```python
from build123d import *

# Parameters (mm, degrees)
RESSALTO_EXTRUS_O1_DEPTH = 20
CORTE_EXTRUS_O1_DEPTH    = 118
CORTE_EXTRUS_O2_DEPTH    = 137.674796506
ESBO_O4_R                = 11.969366969
CORTE_EXTRUS_O3_DEPTH    = 137.674796506


with BuildPart() as part:
    # Esboço1 → Ressalto-extrusão1 (new body)
    with BuildSketch(Plane.XY):
        Polygon((0, 0), (0, 18), (8, 18), (8, 8), (126, 8), (126, 18), (134, 18), (134, 0), align=None)
    extrude(amount=RESSALTO_EXTRUS_O1_DEPTH)

    # Esboço2 → Corte-extrusão1 (cut)
    with BuildSketch(Plane(origin=(8, 0, 0), x_dir=(0, 0, -1), z_dir=(1, 0, 0))):
        with BuildLine():
            Line((-20, 8), (0, 8))
            ThreePointArc((0, 8), (-10, 6.284271247), (-20, 8))
        make_face()
    extrude(amount=CORTE_EXTRUS_O1_DEPTH, mode=Mode.SUBTRACT)

    # Esboço3 → Corte-extrusão2 (cut, through all)
    with BuildSketch(Plane(origin=(0, 0, 0), x_dir=(-1, 0, 0), z_dir=(0, 0, -1))):
        with BuildLine():
            Line((-8, 18), (-7.073837994, 18))
            ThreePointArc((-7.073837994, 18), (-7.767965092, 13.021398611), (-8, 8))
            Line((-8, 8), (-8, 18))
        make_face()
        with BuildLine():
            Line((-126, 8), (-126, 18))
            Line((-126, 18), (-126.926162006, 18))
            ThreePointArc((-126.926162006, 18), (-126.232034908, 13.021398611), (-126, 8))
        make_face()
    extrude(amount=-CORTE_EXTRUS_O2_DEPTH, mode=Mode.SUBTRACT)

    # Esboço4 → Corte-extrusão3 (cut, through all)
    with BuildSketch(Plane.ZY):
        with Locations((10, 27.253795072)):
            Circle(ESBO_O4_R)
    extrude(amount=-CORTE_EXTRUS_O3_DEPTH, mode=Mode.SUBTRACT)


solid = part.part
```
Input: part model. Units: mm. Frame: model coordinates. A direction names the side the tool comes from. Give positions to 0.01 mm unless a question says otherwise; leave off trailing zeros. Write each loop counter-clockwise with the first axis right and the second up, starting at its lowest first coordinate (ties: lowest second). Pieces come first, ordered by that corner, then holes. Notation, with made-up numbers: (-22, 47.5) - (16, 47.5) arc R29 ccw to (16, 84.5) - close; hole circle Ø8 at (85.25, 54). An arc over 180 degrees is marked (long way). Write item = value, one per line. Start each with the question number.
1) Draft query along X for faces 1 (the face through (0, 9, 10)), 2 (the face through (134, 9, 10)), 3 (the face through (126.146, 11.978, 9.86)), 4 (the face through (68, 5, 20)). Return one class per face: pulls with the +X half, pulls with the -X half, needs draft (parallel to the pull), parting line crosses it, or undercut.
2) Pin query (flat end, axial travel): pin 1 (4 mm diameter, centred on x = 101, z = 17.5, fed in from +Y); pin 2 (6 mm diameter, centred on y = 6.5, z = 15.5, fed in from -X); pin 3 (12 mm diameter, centred on x = 20, z = 16.5, fed in from +Y). Return the tip coordinate at first contact, or that it passes through.
3) Reachability of faces 5 (the face through (130.192, 15.285, 9.885)), 6 (the face through (7.854, 11.978, 9.86)), 7 (the face through (66.174, 6.285, 9.857)) from +Z, -Z, +X, -X, +Y, -Y: full face, straight path, thin tool, end or side. Return the list, or none.
4) Material intervals for L1, parallel to X at y = 9.5, z = 18.75; L2, parallel to X at y = 10.25, z = 14; L3, parallel to Y at x = 102.5, z = 16.75, sorted ascending. Write a range as [from, to].
5) Cut plane C-C (x = 61). Return loops of the section in (y, z).
6) Cut plane B-B (z = 12). Return loops of the section in (x, y).
7) Cut plane A-A (y = 9.75). Return loops of the section in (x, z).
8) Cut plane D-D (z = 5.5). Return loops of the section in (x, y), and give its area (3 significant figures).
Answers follow:
q1.face_1 = pulls with the -X half
q1.face_2 = pulls with the +X half
q1.face_3 = undercut
q1.face_4 = needs draft
q2.pin_1 = 7.83
q2.pin_2 = 0
q2.pin_3 = 8
q3.face_5 = +X, -X, +Y
q3.face_6 = +Z, -Z, +Y
q3.face_7 = +Y
q4.L1 = [0, 7.98], [126.02, 134]
q4.L2 = [0, 7.95], [126.05, 134]
q4.L3 = [0, 7.05]
q5.outline = (0, 0) - (8, 0) arc R30 cw to (8, 20) - (0, 20) - close
q6.outline = (0, 0) - (134, 0) - (134, 15.45) - (126.51, 15.45) arc R54.45 ccw to (126, 8) - (126, 6.35) - (8, 6.35) - (8, 8) arc R54.45 ccw to (7.49, 15.45) - (0, 15.45) - close
q7.outline = (0, 0) - (7.97, 0) - (7.97, 20) - (0, 20) - close; (126.03, 0) - (134, 0) - (134, 20) - (126.03, 20) - close
q8.outline = (0, 0) - (134, 0) - (134, 16.16) - (126.62, 16.16) arc R54.45 ccw to (126, 8) - (126, 6.62) - (8, 6.62) - (8, 8) arc R54.45 ccw to (7.38, 16.16) - (0, 16.16) - close
q8.area = 1,040 mm^2
